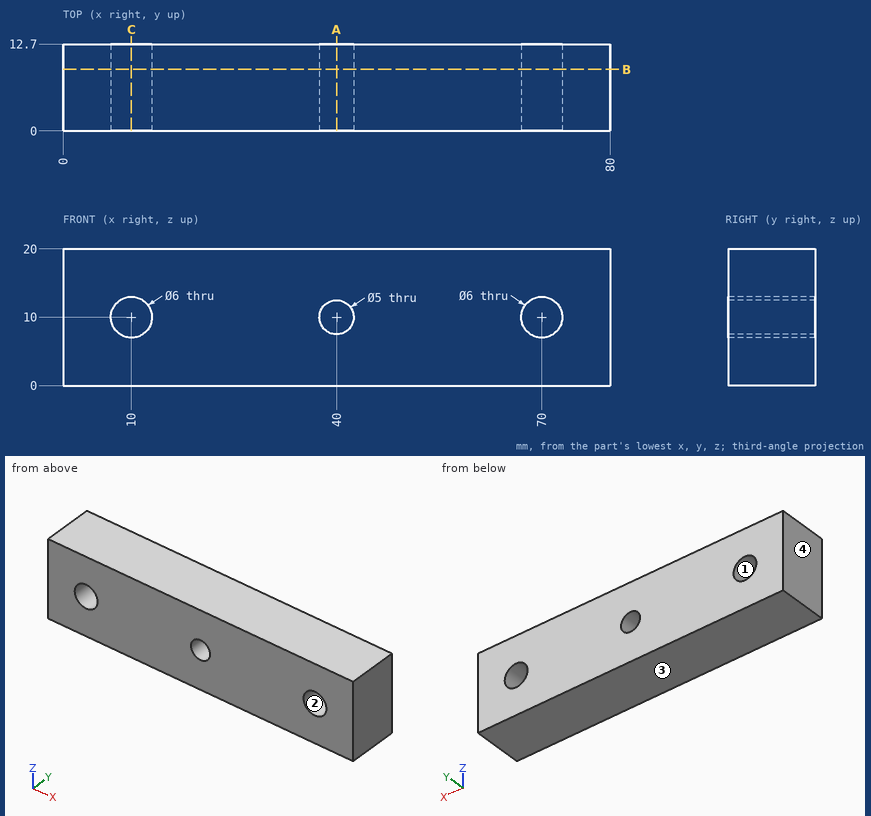
Check sheet for the drawn part. Datum: minimum x, y, z corner. Units: mm. Give positions to 0.01 mm unless a question says otherwise; leave off trailing zeros. Write each loop counter-clockwise with the first axis right and the second up, starting at its lowest first coordinate (ties: lowest second). Pieces come first, ordered by that corner, then holes.
(1) Cross-section at C-C (x = 10). Enter the section's corners in (y, z), plus the area to 3 significant figures.
(2) Cross-section at B-B (y = 9). Enter the section's corners in (x, z), plus the area to 3 significant figures.
(3) Cross-section at A-A (x = 40). Enter the section's corners in (y, z).
(4) Gauge pin test, flat end, axial feed: pin 1 (5 mm diameter, centred on x = 10, z = 10, fed in from -Y) (3 decimals). Record the tip position at first contact, or that the pin passes through.
(5) Material ranges on line 1 (X direction, y = 4.75, z = 10); line 2 (X direction, y = 6.25, z = 10.75); line 3 (Z direction, x = 40.5, y = 4.5), recorded low to high.
(6) Mould release check, pull along Z, two halves, no side actions. Record for the marked faces 1, 2, 3 and 4: +Z half, -Z half, draft (parallel to the pull), parting line (faces both ways), or undercut.
Worked out:
1. outline: (0, 0) - (12.7, 0) - (12.7, 7) - (0, 7) - close; (0, 13) - (12.7, 13) - (12.7, 20) - (0, 20) - close
1. area: 178 mm2
2. outline: (0, 0) - (80, 0) - (80, 20) - (0, 20) - close; hole circle Ø6 at (10, 10); hole circle Ø5 at (40, 10); hole circle Ø6 at (70, 10)
2. area: 1,520 mm2
3. outline: (0, 0) - (12.7, 0) - (12.7, 7.5) - (0, 7.5) - close; (0, 12.5) - (12.7, 12.5) - (12.7, 20) - (0, 20) - close
4. pin 1: passes through
5. line 1: x = 0 to 7, 13 to 37.5, 42.5 to 67, 73 to 80
5. line 2: x = 0 to 7.1, 12.9 to 37.62, 42.38 to 67.1, 72.9 to 80
5. line 3: z = 0 to 7.55, 12.45 to 20
6. face 1: undercut
6. face 2: undercut
6. face 3: -Z half
6. face 4: draft
